Source: CAD feature listing. Evaluate the final solid. Frame: model axes, mm. A direction names the side the tool comes from. Coordinates: 2 decimals unless noted, no trailing zeros. Loops run counter-clockwise (first coordinate to the right, second up) from the corner with the lowest first, then second, coordinate; pieces in that order, holes last.
Item 1: Pin query (flat end, axial travel): pin 1 Ø11.5 at (y, z) = (0, 0) entering from -X; pin 2 Ø1.5 at (x, z) = (-2, -9) entering from +Y; pin 3 Ø2 at (x, z) = (1.5, -20) entering from -Y; pin 4 Ø4 at (y, z) = (0.5, -1) entering from -X (3 decimals). Return the tip coordinate at first contact, or that it passes through.
Item 2: Line query: probe 1 along Z at (x, y) = (-0.75, -3.5); probe 2 along X at (y, z) = (0.5, -47.5); probe 3 along Y at (x, z) = (-1.25, -67). Output: solid intervals per line, ascending.
Item 3: Pull-direction query (Y, two-part tool) for faces 1 (the cylindrical face through (-0.042, 4.115, -29.952)), 2 (the cylindrical face through (0.042, -4.115, -29.952)), 3 (the cylindrical face through (-3.507, -0.22, -78.997)); classes: +Y half, -Y half, draft (parallel to the pull), parting line (faces both ways), or undercut.
Item 4: Reachability of faces 4 (the cylindrical face through (-3.493, -2.694, -9.699)), 5 (the flat face through (0.042, -7.605, -50.095)), 6 (the cylindrical face through (3.7, -7.41, -50.64)), 7 (the flat face through (3, 0, -34)) from +Z, -Z, +X, -X, +Y, -Y: full face, straight path, thin tool, end or side. Return the list, or none.
Item 5: Section query B-B, the plane y = 0. State how many separate pieces and enclosed holes the cut face has, then the cut area to 3 significant figures.
Item 6: Section query A-A, the plane x = 0. Return the cut outline in (y, z), then the cut area to 3 significant figures.
```python
from build123d import *

# Parameters (mm, degrees)
F0_R     = 5.1
F1_DEPTH = 4
F2_R     = 5.1
F3_DEPTH = 1
F4_R     = 30
F5_R     = 5
F6_R     = 5
F7_R     = 30
F8_R     = 1
F9_R     = 1


# Not quite as in the source:
# - a pattern or mirror of a feature is missing from the dataset's text; its kind, count and spacing are read off the source's solid


with BuildPart() as f1:
    # F0 (on Right) → F1 (new body, symmetric)
    with BuildSketch(Plane.YZ):
        with BuildLine():
            ThreePointArc((4, -10.3542261903), (9.1545070867, -6.2773402011), (11.1, 0))
            ThreePointArc((11.1, 0), (-6.2773402011, 9.1545070867), (-4, -10.3542261903))
            ThreePointArc((-4, -10.3542261903), (0, -11.1), (4, -10.3542261903))
        make_face()
        Circle(F0_R, mode=Mode.SUBTRACT)
        with BuildLine():
            ThreePointArc((4, -10.3542261903), (0, -11.1), (-4, -10.3542261903))
            Line((-4, -10.3542261903), (-4, -30))
            Line((-4, -30), (-10.8271665456, -68.0577166546))
            ThreePointArc((-10.8271665456, -68.0577166546), (0, -59), (10.8271665456, -68.0577166546))
            Line((10.8271665456, -68.0577166546), (4, -30))
            Line((4, -30), (4, -10.3542261903))
        make_face()
        with BuildLine():
            ThreePointArc((10.8271665456, -68.0577166546), (0, -59), (-10.8271665456, -68.0577166546))
            ThreePointArc((-10.8271665456, -68.0577166546), (-0.9749789737, -80.9567064395), (11, -70))
            ThreePointArc((11, -70), (10.9567064395, -69.0250210263), (10.8271665456, -68.0577166546))
        make_face()
        with Locations((0, -70)):
            Circle(F0_R, mode=Mode.SUBTRACT)
    extrude(amount=F1_DEPTH, both=True)

    # F2 (on face) → F3 (cut)
    with BuildSketch(Plane.YZ.offset(4)):
        with BuildLine():
            Line((2, -30.1779693522), (2, -8.877499648))
            ThreePointArc((2, -8.877499648), (0, 9.1), (-2, -8.877499648))
            Line((-2, -8.877499648), (-2, -30.1779693522))
            Line((-2, -30.1779693522), (-8.85859081, -68.410859081))
            ThreePointArc((-8.85859081, -68.410859081), (0, -79), (8.85859081, -68.410859081))
            Line((8.85859081, -68.410859081), (2, -30.1779693522))
        make_face()
        with Locations((0, -70)):
            Circle(F2_R, mode=Mode.SUBTRACT)
        Circle(F2_R, mode=Mode.SUBTRACT)
    f3 = extrude(amount=-F3_DEPTH, mode=Mode.SUBTRACT)

    # F3_copies: F3 across plane
    add(f3.mirror(Plane(origin=(0, 0, 0), x_dir=(0, 0, -1), z_dir=(-1, 0, 0))), mode=Mode.SUBTRACT)

    # F4
    f4_edges = [f1.edges().sort_by_distance(p)[0] for p in [
        (0, -4, -30),
        (0, 4, -30),
    ]]
    fillet(f4_edges, radius=F4_R)

    # F5
    f5_edges = [f1.edges().sort_by_distance(p)[0] for p in [
        (0, -4, -10.354226),
        (0, 4, -10.354226),
    ]]
    fillet(f5_edges, radius=F5_R)

    # F6
    f6_edges = [f1.edges().sort_by_distance(p)[0] for p in [
        (3.5, -2, -8.8775),
        (3.5, 2, -8.8775),
        (-3.5, 2, -8.8775),
        (-3.5, -2, -8.8775),
    ]]
    fillet(f6_edges, radius=F6_R)

    # F7
    f7_edges = [f1.edges().sort_by_distance(p)[0] for p in [
        (-3.5, 2, -30.177969),
        (-3.5, -2, -30.177969),
        (3.5, 2, -30.177969),
        (3.5, -2, -30.177969),
    ]]
    fillet(f7_edges, radius=F7_R)

    # F8
    f8_edges = [f1.edges().sort_by_distance(p)[0] for p in [
        (4, 0, 11.1),
        (4, -4.585526, -11.001677),
        (4, -4, -20.339996),
        (4, -4.118073, -29.989493),
        (4, -7.649265, -50.342656),
        (4, 0, -81),
        (4, 7.649265, -50.342656),
        (4, 4.118073, -29.989493),
        (4, 4, -20.339996),
        (4, 4.585526, -11.001677),
    ]]
    fillet(f8_edges, radius=F8_R)

    # F9
    f9_edges = [f1.edges().sort_by_distance(p)[0] for p in [
        (-4, 0, 11.1),
        (-4, -4.585526, -11.001677),
        (-4, 4.585526, -11.001677),
        (-4, 4, -20.339996),
        (-4, -4, -20.339996),
        (-4, -4.118073, -29.989493),
        (-4, -7.649265, -50.342656),
        (-4, 0, -81),
        (-4, 7.649265, -50.342656),
        (-4, 4.118073, -29.989493),
    ]]
    fillet(f9_edges, radius=F9_R)


solid = f1.part
```
Verdict:
1. pin 1: stops at x = -3
1. pin 2: stops at y = 7.43
1. pin 3: stops at y = -4
1. pin 4: passes through
2. probe 1: z = -80.43 to -73.71, -66.29 to -3.71, 3.71 to 10.53
2. probe 2: x = -3 to 3
2. probe 3: y = -10.64 to -4.12, 4.12 to 10.64
3. face 1: +Y half
3. face 2: -Y half
3. face 3: undercut
4. face 4: -X
4. face 5: +X, -X, -Y
4. face 6: +X, -Y
4. face 7: +X
5. separate pieces: 3
5. enclosed holes: 0
5. area: 437 mm2
6. outline: (-10.83, -68.06) arc R11 ccw (long way) to (10.83, -68.06) - (4.47, -32.63) arc R30 cw to (4, -27.33) - (4, -13.35) arc R5 cw to (6.2, -9.2) arc R11.1 ccw (long way) to (-6.2, -9.2) arc R5 cw to (-4, -13.35) - (-4, -27.33) arc R30 cw to (-4.47, -32.63) - close; hole circle Ø10.2 at (0, -70); hole circle Ø10.2 at (0, 0)
6. area: 1,180 mm2
